```python
from build123d import *

# Parameters (mm, degrees)
F1_DEPTH = 40
F6_DEPTH = 360
F7_DEPTH = 360
F8_DEPTH = 360
F9_DEPTH = 360


with BuildPart() as f1:
    # F0 (on Top) → F1 (new body)
    with BuildSketch(Plane.XY):
        with BuildLine():
            Line((178.077192, 137.014396), (-161.922808, 137.014396))
            ThreePointArc((-161.922808, 137.014396), (-183.136011, 128.227599), (-191.922808, 107.014396))
            Line((-191.922808, 107.014396), (-191.922808, -232.985604))
            ThreePointArc((-191.922808, -232.985604), (-183.136011, -254.198808), (-161.922808, -262.985604))
            Line((-161.922808, -262.985604), (178.077192, -262.985604))
            ThreePointArc((178.077192, -262.985604), (199.290396, -254.198808), (208.077192, -232.985604))
            Line((208.077192, -232.985604), (208.077192, 107.014396))
            ThreePointArc((208.077192, 107.014396), (199.290396, 128.227599), (178.077192, 137.014396))
        make_face()
    extrude(amount=F1_DEPTH)

    # F2 (on face) → F6 (join)
    with BuildSketch(Plane(origin=(0, 0, 0), x_dir=(1, 0, 0), z_dir=(0, 0, -1))):
        with BuildLine():
            Line((-121.922808, -57.014396), (-141.922808, -57.014396))
            ThreePointArc((-141.922808, -57.014396), (-148.993876, -59.943328), (-151.922808, -67.014396))
            Line((-151.922808, -67.014396), (-151.922808, -87.014396))
            ThreePointArc((-151.922808, -87.014396), (-148.993876, -94.085464), (-141.922808, -97.014396))
            Line((-141.922808, -97.014396), (-121.922808, -97.014396))
            ThreePointArc((-121.922808, -97.014396), (-114.85174, -94.085464), (-111.922808, -87.014396))
            Line((-111.922808, -87.014396), (-111.922808, -67.014396))
            ThreePointArc((-111.922808, -67.014396), (-114.85174, -59.943328), (-121.922808, -57.014396))
        make_face()
    extrude(amount=F6_DEPTH)

    # F5 (on face) → F7 (join)
    with BuildSketch(Plane(origin=(0, 0, 0), x_dir=(1, 0, 0), z_dir=(0, 0, -1))):
        with BuildLine():
            Line((158.077192, -57.014396), (138.077192, -57.014396))
            ThreePointArc((138.077192, -57.014396), (131.006124, -59.943328), (128.077192, -67.014396))
            Line((128.077192, -67.014396), (128.077192, -87.014396))
            ThreePointArc((128.077192, -87.014396), (131.006124, -94.085464), (138.077192, -97.014396))
            Line((138.077192, -97.014396), (158.077192, -97.014396))
            ThreePointArc((158.077192, -97.014396), (165.14826, -94.085464), (168.077192, -87.014396))
            Line((168.077192, -87.014396), (168.077192, -67.014396))
            ThreePointArc((168.077192, -67.014396), (165.14826, -59.943328), (158.077192, -57.014396))
        make_face()
    extrude(amount=F7_DEPTH)

    # F3 (on face) → F8 (join)
    with BuildSketch(Plane(origin=(0, 0, 0), x_dir=(1, 0, 0), z_dir=(0, 0, -1))):
        with BuildLine():
            Line((-121.922808, 222.985604), (-141.922808, 222.985604))
            ThreePointArc((-141.922808, 222.985604), (-148.993876, 220.056672), (-151.922808, 212.985604))
            Line((-151.922808, 212.985604), (-151.922808, 192.985604))
            ThreePointArc((-151.922808, 192.985604), (-148.993876, 185.914536), (-141.922808, 182.985604))
            Line((-141.922808, 182.985604), (-121.922808, 182.985604))
            ThreePointArc((-121.922808, 182.985604), (-114.85174, 185.914536), (-111.922808, 192.985604))
            Line((-111.922808, 192.985604), (-111.922808, 212.985604))
            ThreePointArc((-111.922808, 212.985604), (-114.85174, 220.056672), (-121.922808, 222.985604))
        make_face()
    extrude(amount=F8_DEPTH)

    # F4 (on Top) → F9 (join)
    with BuildSketch(Plane.XY):
        with BuildLine():
            ThreePointArc((128.077192, -212.985604), (131.006124, -220.056672), (138.077192, -222.985604))
            Line((138.077192, -222.985604), (158.077192, -222.985604))
            ThreePointArc((158.077192, -222.985604), (165.14826, -220.056672), (168.077192, -212.985604))
            Line((168.077192, -212.985604), (168.077192, -192.985604))
            ThreePointArc((168.077192, -192.985604), (165.14826, -185.914536), (158.077192, -182.985604))
            Line((158.077192, -182.985604), (138.077192, -182.985604))
            ThreePointArc((138.077192, -182.985604), (131.006124, -185.914536), (128.077192, -192.985604))
            Line((128.077192, -192.985604), (128.077192, -212.985604))
        make_face()
    extrude(amount=-F9_DEPTH)


solid = f1.part
```
The model under review builds one solid part; all positions refer to its coordinate system, in mm. A direction names the side the tool comes from. Round coordinates to 2 decimals unless told otherwise and drop trailing zeros. Write each loop counter-clockwise with the first axis right and the second up, starting at its lowest first coordinate (ties: lowest second). Pieces come first, ordered by that corner, then holes.
(1) We need section B-B on x = -1.5. Give the boundary of the cut face in (y, z).
(2) Mouldability with a two-part tool opening along X and no side actions: class faces 5 (the flat face through (148, 57.014, -177)), 6 (the cylindrical face through (-183.37, -253.96, 19.72)), 7 (the flat face through (128.077, 77, -177)) as +X half, -X half, draft (parallel to the pull), parting line (faces both ways), or undercut.
(3) Machinability: for faces 1 (the flat face through (-132, 97.014, -177)), 2 (the flat face through (128.077, -203, -177)), 3 (the flat face through (-151.923, -203, -177)), 4 (the flat face through (-132, -222.986, -177)), which of the approach directions +Z, -Z, +X, -X, +Y, -Y give a long, thin tool a straight path to every point of the face, cutting with its end or side? Answer none if there is none.
(4) We need section C-C on y = -71. Give the boundary of the cut face in (x, z), and give its area (3 significant figures).
(5) We need section A-A on z = -114. Give the number of separate pieces and of enclosed holes in the cut face, and give its area (3 significant figures).
(6) Wall thickness on L1, parallel to X at y = 73, z = -122.5; L2, parallel to Y at x = 144, z = -338; L3, parallel to Z at x = -110, y = -123.5: over which ranges is each line inside the solid? List them lowest first.
(7) Insertion check: pin 1 (6 mm diameter, centred on x = -135.5, z = -202, fed in from +Y); pin 2 (10 mm diameter, centred on x = 148, z = -229.5, fed in from -Y); pin 3 (10 mm diameter, centred on y = -201, z = -168.5, fed in from +X); pin 4 (12 mm diameter, centred on y = -8.5, z = -2, fed in from -X). Each pin has a flat end and moves straight along its axis. Give the tip position at first contact, or say it passes through.
Findings below:
1. outline: (-262.99, 0) - (137.01, 0) - (137.01, 40) - (-262.99, 40) - close
2. face 5: draft
2. face 6: -X half
2. face 7: undercut
3. face 1: -Z, +X, -X, +Y
3. face 2: -Z, +Y, -Y
3. face 3: -Z, -X, +Y, -Y
3. face 4: -Z, +X, -X, -Y
4. outline: (-191.92, 0) - (208.08, 0) - (208.08, 40) - (-191.92, 40) - close
4. area: 16,000 mm2
5. separate pieces: 4
5. enclosed holes: 0
5. area: 6,060 mm2
6. L1: x = -151.92 to -111.92, 128.08 to 168.08
6. L2: y = -222.99 to -182.99, 57.01 to 97.01
6. L3: z = 0 to 40
7. pin 1: stops at y = 97.01
7. pin 2: stops at y = -222.99
7. pin 3: stops at x = 168.08
7. pin 4: stops at x = -191.92
